Check sheet for the modelled part. Datum: model origin and axes. Units: mm. Face numbers are marked on the shaded views. A direction names the side the tool comes from. Give positions to 0.01 mm unless a question says otherwise; leave off trailing zeros. Loops run counter-clockwise (first coordinate to the right, second up) from the corner with the lowest first, then second, coordinate; pieces in that order, holes last. Notation, with made-up numbers: M 48,-14 L 75,-14 A23 cw 75,14 Z; hole C -20.5,72 d5. An arc over 180 degrees is marked long. Use one line per item in the form item = value.
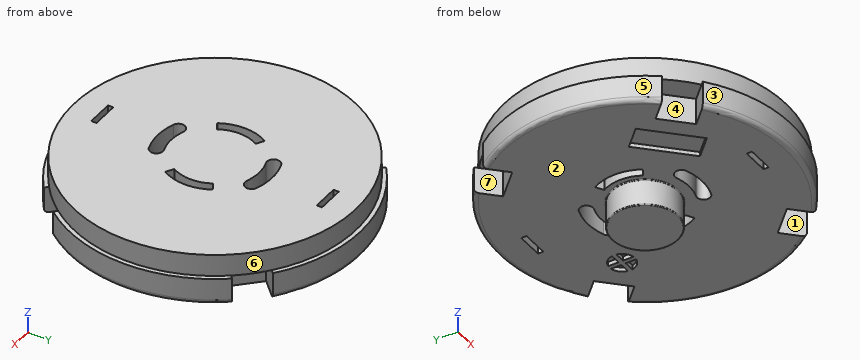
from build123d import *

# Parameters (mm, degrees)
SKETCH1_R           = 16.5
BOSS_EXTRUDE1_DEPTH = 3
SKETCH2_R           = 3.75
BOSS_EXTRUDE2_DEPTH = 3
CUT_EXTRUDE1_DEPTH  = 4
CIRPATTERN1_COUNT   = 4
SKETCH4_R           = 16
BOSS_EXTRUDE3_DEPTH = 2.5
CUT_EXTRUDE2_DEPTH  = 6.5
CIRPATTERN2_COUNT   = 2
CUT_EXTRUDE3_DEPTH  = 6.5
CIRPATTERN3_COUNT   = 2
SKETCH8_R           = 1.45
CUT_EXTRUDE4_DEPTH  = 0.5
SKETCH9_W           = 0.5
SKETCH9_H           = 2.9
EXTRUDE_THIN1_DEPTH = 0.5
SKETCH10_W          = 2.9
SKETCH10_H          = 0.5
EXTRUDE_THIN2_DEPTH = 0.5
SKETCH11_W          = 3
SKETCH11_H          = 0.6
CUT_EXTRUDE5_DEPTH  = 6.5
CIRPATTERN4_COUNT   = 2
FILLET1_R           = 0.1
FILLET2_R           = 0.5


with BuildPart() as part:
    # Sketch1 → Boss-Extrude1 (new body)
    with BuildSketch(Plane.XY):
        Circle(SKETCH1_R)
    extrude(amount=-BOSS_EXTRUDE1_DEPTH)

    # Sketch2 → Boss-Extrude2 (add)
    with BuildSketch(Plane(origin=(0, 0, -3), x_dir=(-1, 0, 0), z_dir=(0, 0, -1))):
        Circle(SKETCH2_R)
    extrude(amount=BOSS_EXTRUDE2_DEPTH)

    # Sketch3 → Cut-Extrude1 (cut, through all)
    with BuildSketch(Plane(origin=(0, 0, -3), x_dir=(-1, 0, 0), z_dir=(0, 0, -1))):
        Polygon((10.253048327, 13.081475452), (8.131727984, 10.960155108), (10.960155108, 8.131727984), (13.081475452, 10.253048327), align=None)
    cut_extrude1 = extrude(amount=-CUT_EXTRUDE1_DEPTH, mode=Mode.SUBTRACT)

    # CirPattern1: Cut-Extrude1 ×4 about axis
    cirpattern1_axis = Axis((0, 0, 0), (0, 0, 1))
    for i in range(1, CIRPATTERN1_COUNT):
        add(cut_extrude1.rotate(cirpattern1_axis, i * 360 / CIRPATTERN1_COUNT), mode=Mode.SUBTRACT)

    # Sketch4 → Boss-Extrude3 (add)
    with BuildSketch(Plane.XY):
        Circle(SKETCH4_R)
    extrude(amount=BOSS_EXTRUDE3_DEPTH)

    # Sketch6 → Cut-Extrude2 (cut, through all)
    with BuildSketch(Plane(origin=(0, 0, -3), x_dir=(-1, 0, 0), z_dir=(0, 0, -1))):
        with BuildLine():
            Line((-4.67653718, 2.7), (-3.810511777, 2.2))
            ThreePointArc((-3.810511777, 2.2), (-4.4, 0), (-3.810511777, -2.2))
            Line((-3.810511777, -2.2), (-4.67653718, -2.7))
            ThreePointArc((-4.67653718, -2.7), (-5.4, 0), (-4.67653718, 2.7))
        make_face()
    cut_extrude2 = extrude(amount=-CUT_EXTRUDE2_DEPTH, mode=Mode.SUBTRACT)

    # CirPattern2: Cut-Extrude2 ×2 about axis
    cirpattern2_axis = Axis((0, 0, 0), (0, 0, 1))
    for i in range(1, CIRPATTERN2_COUNT):
        add(cut_extrude2.rotate(cirpattern2_axis, i * 360 / CIRPATTERN2_COUNT), mode=Mode.SUBTRACT)

    # Sketch7 → Cut-Extrude3 (cut, through all)
    with BuildSketch(Plane(origin=(0, 0, -3), x_dir=(-1, 0, 0), z_dir=(0, 0, -1))):
        with BuildLine():
            ThreePointArc((2.223130932, 6.108002035), (0, 6.5), (-2.223130932, 6.108002035))
            ThreePointArc((-2.223130932, 6.108002035), (-2.67138529, 5.146717462), (-1.710100717, 4.698463104))
            ThreePointArc((-1.710100717, 4.698463104), (0, 5), (1.710100717, 4.698463104))
            ThreePointArc((1.710100717, 4.698463104), (2.67138529, 5.146717462), (2.223130932, 6.108002035))
        make_face()
    cut_extrude3 = extrude(amount=-CUT_EXTRUDE3_DEPTH, mode=Mode.SUBTRACT)

    # CirPattern3: Cut-Extrude3 ×2 about axis
    cirpattern3_axis = Axis((0, 0, 0), (0, 0, 1))
    for i in range(1, CIRPATTERN3_COUNT):
        add(cut_extrude3.rotate(cirpattern3_axis, i * 360 / CIRPATTERN3_COUNT), mode=Mode.SUBTRACT)

    # Sketch8 → Cut-Extrude4 (cut)
    with BuildSketch(Plane(origin=(0, 0, -3), x_dir=(-1, 0, 0), z_dir=(0, 0, -1))):
        with Locations((-7.071067812, 7.071067812)):
            Circle(SKETCH8_R)
        Polygon((8.485281374, -3.535533906), (3.535533906, -8.485281374), (5.656854249, -10.606601718), (10.606601718, -5.656854249), align=None)
    extrude(amount=-CUT_EXTRUDE4_DEPTH, mode=Mode.SUBTRACT)

    # Sketch9 → Extrude-Thin1 (add)
    with BuildSketch(Plane(origin=(0, 0, -2.5), x_dir=(-1, 0, 0), z_dir=(0, 0, -1))):
        with Locations((-7.071067812, 7.071067812)):
            Rectangle(SKETCH9_W, SKETCH9_H)
    extrude(amount=EXTRUDE_THIN1_DEPTH)

    # Sketch10 → Extrude-Thin2 (add)
    with BuildSketch(Plane(origin=(0, 0, -2.5), x_dir=(-1, 0, 0), z_dir=(0, 0, -1))):
        with Locations((-7.071067812, 7.071067812)):
            Rectangle(SKETCH10_W, SKETCH10_H)
    extrude(amount=EXTRUDE_THIN2_DEPTH)

    # Sketch11 → Cut-Extrude5 (cut, through all)
    with BuildSketch(Plane(origin=(0, 0, -3), x_dir=(-1, 0, 0), z_dir=(0, 0, -1))):
        with Locations((0, 12.8)):
            Rectangle(SKETCH11_W, SKETCH11_H)
    cut_extrude5 = extrude(amount=-CUT_EXTRUDE5_DEPTH, mode=Mode.SUBTRACT)

    # CirPattern4: Cut-Extrude5 ×2 about axis
    cirpattern4_axis = Axis((0, 0, 0), (0, 0, 1))
    for i in range(1, CIRPATTERN4_COUNT):
        add(cut_extrude5.rotate(cirpattern4_axis, i * 360 / CIRPATTERN4_COUNT), mode=Mode.SUBTRACT)

    # Fillet1
    fillet1_edges = [part.edges().sort_by_distance(p)[0] for p in [
        (3.75, 0, -3),
        (3.75, 0, -6),
    ]]
    fillet(fillet1_edges, radius=FILLET1_R)

    # Fillet2
    fillet2_edges = [part.edges().sort_by_distance(p)[0] for p in [
        (-16.5, 0, -3),
        (0, -16.5, -3),
        (16.5, 0, -3),
        (0, 16.5, -3),
    ]]
    fillet(fillet2_edges, radius=FILLET2_R)


solid = part.part
1) Scan lines: line 1 (Y direction, x = -2, z = -2); line 2 (Y direction, x = 2.5, z = -0.75); line 3 (X direction, y = 1, z = -1.25). Record each from-to range of solid material in increasing order.
Evaluation:
line_1 = -16.38 to -6.18, -4.65 to 4.65, 6.18 to 16.38
line_2 = -16.31 to -5.93, -4.88 to 4.88, 5.93 to 16.31
line_3 = -16.47 to -5.31, -4.28 to 4.28, 5.31 to 16.47
2) Section check B-B (x = 0). State how many separate pieces and enclosed holes the cut face has, then the cut area to 3 significant figures.
Evaluation:
separate_pieces = 5
enclosed_holes = 0
area = 178 mm^2
3) Set-up check for the marked faces 4, 5, 6 and 7: record each of +Z, -Z, +X, -X, +Y, -Y from which the full face is reachable in a straight line by a thin tool's end or side.
Evaluation:
face_4 = -Z
face_5 = +Z, -Z, -X
face_6 = +Z
face_7 = -Z, -X
4) Release check for a two-part mould opening along X. For the marked faces 1, 2 and 3 record: pulls with the +X half, pulls with the -X half, needs draft (parallel to the pull), parting line crosses it, or undercut.
Evaluation:
face_1 = undercut
face_2 = needs draft
face_3 = parting line crosses it
5) Section check C-C (z = 1). Record the cut outline in (x, y), then the cut area to 3 significant figures.
Evaluation:
outline = C 0,0 d32; hole M -4.68,-2.7 L -3.81,-2.2 A4.4 cw -3.81,2.2 L -4.68,2.7 A5.4 ccw Z; hole M -2.22,-6.11 A6.5 ccw 2.22,-6.11 A0.75 ccw 1.71,-4.7 A5 cw -1.71,-4.7 A0.75 ccw Z; hole M -2.22,6.11 A0.75 ccw -1.71,4.7 A5 cw 1.71,4.7 A0.75 ccw 2.22,6.11 A6.5 ccw Z; hole M -1.5,-13.1 L 1.5,-13.1 L 1.5,-12.5 L -1.5,-12.5 Z; hole M -1.5,12.5 L 1.5,12.5 L 1.5,13.1 L -1.5,13.1 Z; hole M 3.81,-2.2 L 4.68,-2.7 A5.4 ccw 4.68,2.7 L 3.81,2.2 A4.4 cw Z
area = 775 mm^2
6) Section check A-A (y = 0). Record the cut outline in (x, z).
Evaluation:
outline = M -16.5,-2.5 A0.5 ccw -16,-3 L -5.4,-3 L -5.4,2.5 L -16,2.5 L -16,0 L -16.5,0 Z; M -4.4,-3 L -3.85,-3 A0.1 cw -3.75,-3.1 L -3.75,-5.9 A0.1 ccw -3.65,-6 L 3.65,-6 A0.1 ccw 3.75,-5.9 L 3.75,-3.1 A0.1 cw 3.85,-3 L 4.4,-3 L 4.4,2.5 L -4.4,2.5 Z; M 5.4,-3 L 16,-3 A0.5 ccw 16.5,-2.5 L 16.5,0 L 16,0 L 16,2.5 L 5.4,2.5 Z
7) Depth check by flat-ended pin: pin 1 Ø5 at (x, y) = (10, -9.5) entering from -Z; pin 2 Ø0.5 at (y, z) = (13, -1) entering from +X; pin 3 Ø0.9 at (x, z) = (0.5, -1.5) entering from -Y; pin 4 Ø2 at (y, z) = (-3, 0) entering from -X. Enter the tip coordinate at first touch or a pass-through.
Evaluation:
pin_1 = -3
pin_2 = 10.17
pin_3 = -16.5
pin_4 = -16.38
